from build123d import *

# Parameters (mm, degrees)
SKETCH_1_W          = 58.5
SKETCH_1_H          = 42
EXTRUDE_1_DEPTH     = 123
CUT_EXTRUDE_1_DEPTH = 120
SKETCH_3_W          = 58.5
SKETCH_3_H          = 123
CUT_EXTRUDE_2_DEPTH = 4
SKETCH_4_W          = 52.5
SKETCH_4_H          = 120
CUT_EXTRUDE_3_DEPTH = 1
SKETCH_5_W          = 58.5
SKETCH_5_H          = 38
CUT_EXTRUDE_4_DEPTH = 10
SKETCH_6_W          = 7
SKETCH_6_H          = 113
EXTRUDE_2_DEPTH     = 5
SKETCH_10_W         = 3
SKETCH_10_H         = 20
CUT_EXTRUDE_5_DEPTH = 33
HOLE_WIZARD_2_D     = 3.5
SKETCH_13_W         = 7
SKETCH_13_H         = 113
EXTRUDE_3_DEPTH     = 5
HOLE_WIZARD_3_D     = 3.5
SKETCH_17_W         = 7
SKETCH_17_H         = 35
SKETCH_17_H_2       = 30
CUT_EXTRUDE_6_DEPTH = 5
SKETCH_18_W         = 3
SKETCH_18_H         = 20
EXTRUDE_4_DEPTH     = 5
SKETCH_19_W         = 28
SKETCH_19_H         = 20
CUT_EXTRUDE_7_DEPTH = 2
FILLET_3_R          = 2
SKETCH_21_W         = 33
SKETCH_21_H         = 30
EXTRUDE_6_DEPTH     = 30
SKETCH_22_W         = 15
SKETCH_22_H         = 33
EXTRUDE_7_DEPTH     = 30
SKETCH_24_W         = 18
SKETCH_24_H         = 20
CUT_EXTRUDE_8_DEPTH = 30
HOLE_WIZARD_4_D     = 23
HOLE_WIZARD_4_DEPTH = 15
SKETCH_27_W         = 15
SKETCH_27_H         = 60
EXTRUDE_8_DEPTH     = 5
SKETCH_28_W         = 45
SKETCH_28_H         = 3
EXTRUDE_9_DEPTH     = 15
SKETCH_29_W         = 14.5
SKETCH_29_H         = 30
SKETCH_29_W_2       = 12.5
EXTRUDE_10_DEPTH    = 15
FILLET_6_R          = 20
SKETCH_30_W         = 2
SKETCH_30_H         = 22
CUT_EXTRUDE_9_DEPTH = 102.775488208


with BuildPart() as part:
    # 草图1 → 凸台-拉伸1 (new body)
    with BuildSketch(Plane(origin=(0, 0, 0), x_dir=(1, 0, 0), z_dir=(0, 1, 0))):
        with Locations((29.25, 21)):
            Rectangle(SKETCH_1_W, SKETCH_1_H)
    extrude(amount=EXTRUDE_1_DEPTH)

    # 草图2 → 切除-拉伸1 (cut)
    with BuildSketch(Plane(origin=(0, 123, 0), x_dir=(1, 0, 0), z_dir=(0, 1, 0))):
        Polygon((3, 3), (4.178571429, 3), (54.321428571, 39), (3, 39), align=None)
        Polygon((54.321428571, 39), (4.178571429, 3), (55.5, 3), (55.5, 39), align=None)
    extrude(amount=-CUT_EXTRUDE_1_DEPTH, mode=Mode.SUBTRACT)

    # 草图3 → 切除-拉伸2 (cut)
    with BuildSketch(Plane(origin=(0, 0, -42), x_dir=(-1, 0, 0), z_dir=(0, 0, -1))):
        with Locations((-29.25, 61.5)):
            Rectangle(SKETCH_3_W, SKETCH_3_H)
    extrude(amount=-CUT_EXTRUDE_2_DEPTH, mode=Mode.SUBTRACT)

    # 草图4 → 切除-拉伸3 (cut)
    with BuildSketch(Plane(origin=(0, 0, -3), x_dir=(-1, 0, 0), z_dir=(0, 0, -1))):
        with Locations((-29.25, 63)):
            Rectangle(SKETCH_4_W, SKETCH_4_H)
    extrude(amount=-CUT_EXTRUDE_3_DEPTH, mode=Mode.SUBTRACT)

    # 草图5 → 切除-拉伸4 (cut)
    with BuildSketch(Plane(origin=(0, 123, 0), x_dir=(1, 0, 0), z_dir=(0, 1, 0))):
        with Locations((29.25, 19)):
            Rectangle(SKETCH_5_W, SKETCH_5_H)
    extrude(amount=-CUT_EXTRUDE_4_DEPTH, mode=Mode.SUBTRACT)

    # 草图6 → 凸台-拉伸2 (add)
    with BuildSketch(Plane(origin=(0, 0, -38), x_dir=(-1, 0, 0), z_dir=(0, 0, -1))):
        with Locations((3.5, 56.5)):
            Rectangle(SKETCH_6_W, SKETCH_6_H)
    extrude(amount=-EXTRUDE_2_DEPTH)

    # 草图10 → 切除-拉伸5 (cut)
    with BuildSketch(Plane.XY):
        with Locations((1.5, 10)):
            Rectangle(SKETCH_10_W, SKETCH_10_H)
    extrude(amount=-CUT_EXTRUDE_5_DEPTH, mode=Mode.SUBTRACT)

    # 孔2 (through all)
    with Locations(Plane.XY.offset(-33)):
        with Locations((-3.5, 40.5), (-3.5, 8)):
            Hole(HOLE_WIZARD_2_D / 2)

    # 草图13 → 凸台-拉伸3 (add)
    with BuildSketch(Plane(origin=(0, 0, -38), x_dir=(-1, 0, 0), z_dir=(0, 0, -1))):
        with Locations((-62, 56.5)):
            Rectangle(SKETCH_13_W, SKETCH_13_H)
    extrude(amount=-EXTRUDE_3_DEPTH)

    # 孔3 (through all)
    with Locations(Plane.XY.offset(-33)):
        with Locations((62, 68), (62, 44)):
            Hole(HOLE_WIZARD_3_D / 2)

    # 草图17 → 切除-拉伸6 (cut)
    with BuildSketch(Plane.XY.offset(-33)):
        with Locations((62, 95.5)):
            Rectangle(SKETCH_17_W, SKETCH_17_H)
        with Locations((62, 15)):
            Rectangle(SKETCH_17_W, SKETCH_17_H_2)
    extrude(amount=-CUT_EXTRUDE_6_DEPTH, mode=Mode.SUBTRACT)

    # 草图18 → 凸台-拉伸4 (add)
    with BuildSketch(Plane.XY.offset(-33)):
        with Locations((1.5, 10)):
            Rectangle(SKETCH_18_W, SKETCH_18_H)
    extrude(amount=EXTRUDE_4_DEPTH)

    # 草图19 → 切除-拉伸7 (cut)
    with BuildSketch(Plane.ZY.offset(-3)):
        with Locations((-14, 10)):
            Rectangle(SKETCH_19_W, SKETCH_19_H)
    extrude(amount=-CUT_EXTRUDE_7_DEPTH, mode=Mode.SUBTRACT)

    # 圆角3
    fillet_3_edges = [part.edges().sort_by_distance(p)[0] for p in [
        (5, 20, -1),
    ]]
    fillet(fillet_3_edges, radius=FILLET_3_R)

    # 草图21 → 凸台-拉伸6 (add)
    with BuildSketch(Plane.ZY):
        with Locations((-16.5, 98)):
            Rectangle(SKETCH_21_W, SKETCH_21_H)
    extrude(amount=EXTRUDE_6_DEPTH)

    # 草图22 → 凸台-拉伸7 (add)
    with BuildSketch(Plane(origin=(0, 113, 0), x_dir=(1, 0, 0), z_dir=(0, 1, 0))):
        with Locations((-37.5, 16.5)):
            Rectangle(SKETCH_22_W, SKETCH_22_H)
    extrude(amount=-EXTRUDE_7_DEPTH)

    # 草图24 → 切除-拉伸8 (cut)
    with BuildSketch(Plane.XY):
        with Locations((-23.5, 93)):
            Rectangle(SKETCH_24_W, SKETCH_24_H)
    extrude(amount=-CUT_EXTRUDE_8_DEPTH, mode=Mode.SUBTRACT)

    # 孔4
    with Locations(Plane(origin=(0, 113, 0), x_dir=(1, 0, 0), z_dir=(0, 1, 0))):
        with Locations((-23.5, 16.5)):
            Hole(HOLE_WIZARD_4_D / 2, depth=HOLE_WIZARD_4_DEPTH)

    # 草图27 → 凸台-拉伸8 (add)
    with BuildSketch(Plane(origin=(0, 0, -33), x_dir=(-1, 0, 0), z_dir=(0, 0, -1))):
        with Locations((14.5, 83)):
            Rectangle(SKETCH_27_W, SKETCH_27_H)
    extrude(amount=EXTRUDE_8_DEPTH)

    # 草图28 → 凸台-拉伸9 (add)
    with BuildSketch(Plane(origin=(0, 83, 0), x_dir=(-1, 0, 0), z_dir=(0, -1, 0))):
        with Locations((22.5, 31.5)):
            Rectangle(SKETCH_28_W, SKETCH_28_H)
    extrude(amount=EXTRUDE_9_DEPTH)

    # 草图29 → 凸台-拉伸10 (add)
    with BuildSketch(Plane.XZ.offset(-83)):
        with Locations((-7.25, -15)):
            Rectangle(SKETCH_29_W, SKETCH_29_H)
        with Locations((-38.75, -15)):
            Rectangle(SKETCH_29_W_2, SKETCH_29_H)
    extrude(amount=EXTRUDE_10_DEPTH)

    # 圆角6
    fillet_6_edges = [part.edges().sort_by_distance(p)[0] for p in [
        (-45, 90.5, -33),
    ]]
    fillet(fillet_6_edges, radius=FILLET_6_R)

    # 草图30 → 切除-拉伸9 (cut, through all)
    with BuildSketch(Plane.XZ.offset(-68)):
        Polygon((-10.25, -9.672413793), (-4.25, -23.327586207), (-4.25, -5.5), (-10.25, -5.5), align=None)
        Polygon((-4.25, -27.5), (-4.25, -23.327586207), (-10.25, -9.672413793), (-10.25, -27.5), align=None)
        with Locations((-3.25, -16.5)):
            Rectangle(SKETCH_30_W, SKETCH_30_H)
    extrude(amount=-CUT_EXTRUDE_9_DEPTH, mode=Mode.SUBTRACT)


solid = part.part
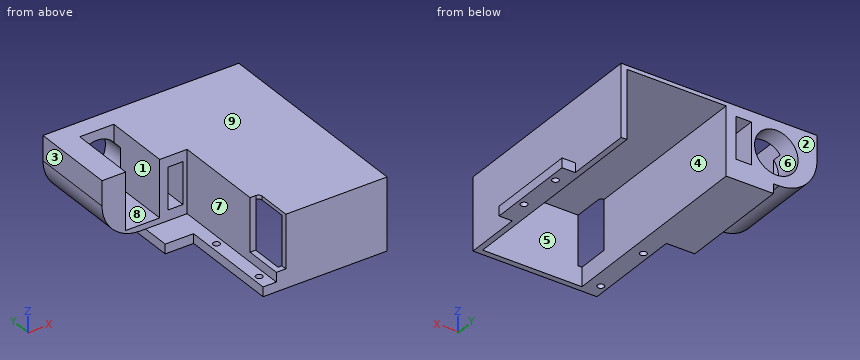
Part model, mm, in its own coordinate system. Face numbers are marked on the shaded views. A direction names the side the tool comes from. Coordinates: 2 decimals unless noted, no trailing zeros. Write each loop counter-clockwise with the first axis right and the second up, starting at its lowest first coordinate (ties: lowest second). Pieces come first, ordered by that corner, then holes. Notation, with made-up numbers: (80.25, 27) - (131.25, 27) arc R12 cw to (131.25, 33) - close; hole circle Ø5 at (56.5, -11.75). An arc over 180 degrees is marked (long way). Put each result on its own line as item: value.
1. 3-axis set-ups, long thin cutter, end or side, ignore diameter. For the marked faces 5, 6, 7, 8 and 9: which of +Z, -Z, +X, -X, +Y, -Y reach the whole face in a straight line?
Final values:
face 5: -Z, +Y
face 6: +Y
face 7: +Z, -X, -Y
face 8: +Z, -Y
face 9: +Z, +X, -X, +Y, -Y
2. Two-plate mould, pull along X, no slides. Class the marked faces 1, 2, 3 and 4: +X half, -X half, draft (parallel to the pull), parting line (faces both ways), or undercut.
Final values:
face 1: undercut
face 2: draft
face 3: -X half
face 4: undercut
3. Band-saw the part on D-D (z = -16.5). Write the cut outline in (x, y), then the cut area to 3 significant figures.
Final values:
outline: (-44.69, 68) - (-32.5, 68) - (-32.5, 98) - (-35, 98) - (-35, 113) - (-44.69, 113) - close; (-14.5, 68) - (-10.25, 68) - (-10.25, 113) - (-12, 113) - (-12, 98) - (-14.5, 98) - close; (-2.25, 68) - (0, 68) - (0, 20) - (3, 20) - (3, 113) - (-2.25, 113) - close; (5, 0) - (58.5, 0) - (58.5, 113) - (55.5, 113) - (55.5, 3) - (5, 3) - close
area: 1,540 mm²
4. Band-saw the part on B-B (y = 44). Write the cut outline in (x, z), then the cut area to 4 significant figures.
Final values:
outline: (-7, -38) - (3, -38) - (3, -2) - (55.5, -2) - (55.5, -38) - (60.25, -38) - (60.25, -33) - (58.5, -33) - (58.5, 0) - (0, 0) - (0, -33) - (-7, -33) - close; (63.75, -38) - (65.5, -38) - (65.5, -33) - (63.75, -33) - close
area: 385.5 mm²
5. Flat gauge pins, fed straight in: pin 1 Ø9 at (y, z) = (91, -9.5) entering from +X; pin 2 Ø5.5 at (x, y) = (3, 14) entering from +Z; pin 3 Ø2 at (x, y) = (19, 89.5) entering from -Z; pin 4 Ø3.5 at (x, y) = (63.5, 46.5) entering from +Z. Where does each tip first touch, or does it go through?
Final values:
pin 1: stops at x = 58.5
pin 2: stops at z = 0
pin 3: stops at z = -2
pin 4: stops at z = -33
6. Probe line 1 along X through (y, z) = (68, -35.15); line 2 along X through (y, z) = (64, -12); line 3 along Y through (x, z) = (62, -34.4). List the from-to ranges inside material, lowest first. Write a range as [from, to].
Final values:
line 1: x = [-22, 3], [55.5, 60.25], [63.75, 65.5]
line 2: x = [0, 3], [55.5, 58.5]
line 3: y = [30, 42.25], [45.75, 66.25], [69.75, 78]
7. Band-saw the part on C-C (x = -23.5). Write the cut outline in (y, z).
Final values:
outline: (68, -33) - (113, -33) - (113, -28) - (103, -28) - (103, -30) - (68, -30) - close; (103, -5) - (113, -5) - (113, 0) - (103, 0) - close
8. Band-saw the part on A-A (x = 62). Write the cut outline in (y, z), then the cut area to 3 significant figures.
Final values:
outline: (30, -38) - (42.25, -38) - (42.25, -33) - (30, -33) - close; (45.75, -38) - (66.25, -38) - (66.25, -33) - (45.75, -33) - close; (69.75, -38) - (78, -38) - (78, -33) - (69.75, -33) - close
area: 205 mm²
